Model file for the job. Use its own axes, mm. Give positions to 0.01 mm unless a question says otherwise; leave off trailing zeros. Write each loop counter-clockwise with the first axis right and the second up, starting at its lowest first coordinate (ties: lowest second). Pieces come first, ordered by that corner, then holes.
```python
from build123d import *

# Parameters (mm, degrees)
BOSS_EXTRUDE1_DEPTH   = 5
CUT_EXTRUDE1_DEPTH    = 1
FILLET1_R             = 2
M3X0_5_TAPPED_HOLE1_D = 2.5
CHAMFER1_SIZE         = 2
FILLET2_R             = 2


with BuildPart() as part:
    # Sketch1 → Boss-Extrude1 (new body)
    with BuildSketch(Plane.XY):
        Polygon((-25, 62.939446367), (7, 62.939446367), (7, -49.560553633), (-59, -49.560553633), (-59, -14.560553633), (-25, -14.560553633), align=None)
        with BuildLine():
            Line((-55.209251079, -23.060553633), (-55.209251079, -41.060553633))
            ThreePointArc((-55.209251079, -41.060553633), (-52.959251079, -43.310553633), (-50.709251079, -41.060553633))
            Line((-50.709251079, -41.060553633), (-50.709251079, -23.060553633))
            ThreePointArc((-50.709251079, -23.060553633), (-52.959251079, -20.810553633), (-55.209251079, -23.060553633))
        make_face(mode=Mode.SUBTRACT)
        with BuildLine():
            Line((-41.108819931, -23.060553633), (-41.108819931, -41.060553633))
            ThreePointArc((-41.108819931, -41.060553633), (-38.858819931, -43.310553633), (-36.608819931, -41.060553633))
            Line((-36.608819931, -41.060553633), (-36.608819931, -23.060553633))
            ThreePointArc((-36.608819931, -23.060553633), (-38.858819931, -20.810553633), (-41.108819931, -23.060553633))
        make_face(mode=Mode.SUBTRACT)
    extrude(amount=BOSS_EXTRUDE1_DEPTH)

    # Sketch5 → Cut-Extrude1 (cut)
    with BuildSketch(Plane.XY.offset(5)):
        with BuildLine():
            Line((-2, 42.249819041), (-2, 23.249819041))
            Line((-2, 23.249819041), (0, 23.249819041))
            Line((0, 23.249819041), (0, 42.249819041))
            ThreePointArc((0, 42.249819041), (2, 44.249819041), (4, 42.249819041))
            Line((4, 42.249819041), (4, -7.750180959))
            Line((4, -7.750180959), (-6, -7.750180959))
            Line((-6, -7.750180959), (-6, 42.249819041))
            ThreePointArc((-6, 42.249819041), (-4, 44.249819041), (-2, 42.249819041))
        make_face()
    extrude(amount=-CUT_EXTRUDE1_DEPTH, mode=Mode.SUBTRACT)

    # Fillet1
    fillet1_edges = [part.edges().sort_by_distance(p)[0] for p in [
        (4, -7.750180959, 4.5),
        (-6, -7.750180959, 4.5),
    ]]
    fillet(fillet1_edges, radius=FILLET1_R)

    # M3x0.5 Tapped Hole1 (through all)
    with Locations(Plane.XY.offset(4)):
        with Locations((-4, 18.542431445), (2, 21.630678546), (2.034899716, 13.630754671), (-4.025360665, 10.542471642), (2.452029153, 5.630754671), (-3.630206533, 2.552236776), (2.358171393, -2.36869473), (-3.536291388, -5.447211951)):
            Hole(M3X0_5_TAPPED_HOLE1_D / 2)

    # Chamfer1
    chamfer1_edges = [part.edges().sort_by_distance(p)[0] for p in [
        (-25, 62.939446367, 2.5),
        (7, 62.939446367, 2.5),
        (7, -49.560553633, 2.5),
        (-59, -49.560553633, 2.5),
        (-59, -14.560553633, 2.5),
        (7, 6.689446367, 5),
    ]]
    chamfer(chamfer1_edges, length=CHAMFER1_SIZE)

    # Fillet2
    fillet2_edges = [part.edges().sort_by_distance(p)[0] for p in [
        (-25, -14.560553633, 2.5),
    ]]
    fillet(fillet2_edges, radius=FILLET2_R)


solid = part.part
```
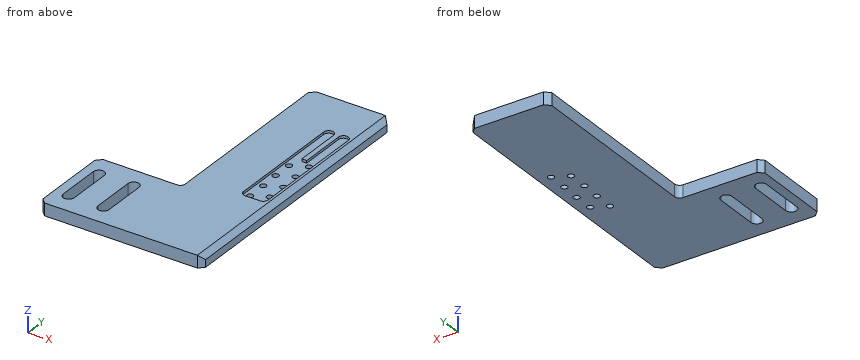
1. Slice it at C-C, the plane y = 0. Write the cut outline in (x, z).
Calculated:
outline: (-25, 0) - (7, 0) - (7, 3) - (5, 5) - (4, 5) - (4, 4) - (-6, 4) - (-6, 5) - (-25, 5) - close
2. Slice it at A-A, the plane y = -40. Write the cut outline in (x, z), and give its area (3 significant figures).
Calculated:
outline: (-59, 0) - (-55.21, 0) - (-55.21, 5) - (-59, 5) - close; (-50.71, 0) - (-41.11, 0) - (-41.11, 5) - (-50.71, 5) - close; (-36.61, 0) - (7, 0) - (7, 3) - (5, 5) - (-36.61, 5) - close
area: 283 mm2
3. Pin check, flat tips, straight feed: P1, Ø0.5, axis at y = 36.5, z = 4.5, coming from the -X side; P2, Ø1.1, axis at y = 24.5, z = 4.5, coming from the +X side; P3, Ø1.5, axis at x = -3.54, y = -5.45, coming from the +Z side; P4, Ø3, axis at y = -16, z = 1, coming from the -X side. Stop position of each tip, or through.
Calculated:
P1: stops at x = -25
P2: stops at x = 6.05
P3: passes through
P4: stops at x = -59
4. Probe probe 1 along X at (y, z) = (-37.5, 1.25); probe 2 along X at (y, z) = (32, 4.4); probe 3 along Y at (x, z) = (2, 2.55). List the from-to ranges inside material, lowest first.
Calculated:
probe 1: x = -59 to -55.21, -50.71 to -41.11, -36.61 to 7
probe 2: x = -25 to -6, -2 to 0, 4 to 5.6
probe 3: y = -49.56 to -3.57, -1.17 to 4.47, 6.8 to 12.38, 14.88 to 20.38, 22.88 to 62.94
5. Slice it at B-B, the plane y = 34. Write the cut outline in (x, z), and give its area (3 significant figures).
Calculated:
outline: (-25, 0) - (7, 0) - (7, 3) - (5, 5) - (4, 5) - (4, 4) - (0, 4) - (0, 5) - (-2, 5) - (-2, 4) - (-6, 4) - (-6, 5) - (-25, 5) - close
area: 150 mm2
